The model under review builds one solid part; all positions refer to its coordinate system, in mm. Face numbers are marked on the shaded views. A direction names the side the tool comes from. Round coordinates to 2 decimals unless told otherwise and drop trailing zeros. Order: outer loops, then holes, each group sorted by start corner. A loop starts at its lowest first (then second) coordinate and runs counter-clockwise, first axis right, second up.
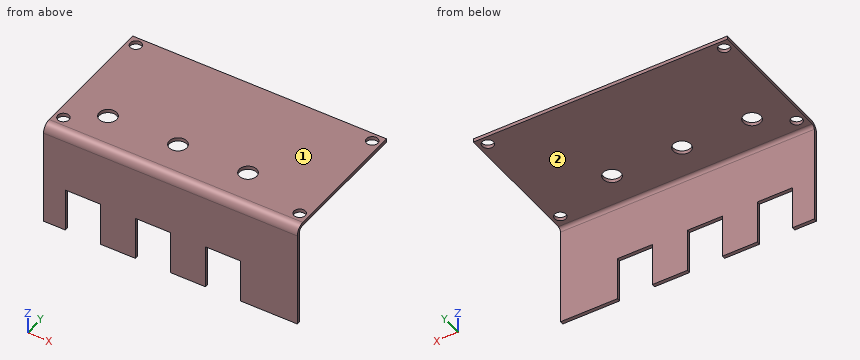
```python
from build123d import *

# Parameters (mm, degrees)
F1_DEPTH = 72.5
F2_W     = 20
F2_H     = 25
F3_DEPTH = 25
F4_R     = 5
F5_DEPTH = 25
F6_R     = 3.25
F7_DEPTH = 25


with BuildPart() as f1:
    # F0 (on Right) → F1 (new body, symmetric)
    with BuildSketch(Plane.YZ):
        with BuildLine():
            Line((34.471770674, 53.4658672512), (34.471770674, 55.4658672512))
            Line((34.471770674, 55.4658672512), (-40.528229326, 55.4658672512))
            ThreePointArc((-40.528229326, 55.4658672512), (-44.0637632319, 54.0014011571), (-45.528229326, 50.4658672512))
            Line((-45.528229326, 50.4658672512), (-45.528229326, -4.5341327488))
            Line((-45.528229326, -4.5341327488), (-43.528229326, -4.5341327488))
            Line((-43.528229326, -4.5341327488), (-43.528229326, 51.4658672512))
            ThreePointArc((-43.528229326, 51.4658672512), (-42.9424428884, 52.8800808135), (-41.528229326, 53.4658672512))
            Line((-41.528229326, 53.4658672512), (34.471770674, 53.4658672512))
        make_face()
    extrude(amount=F1_DEPTH, both=True)

    # F2 (on face) → F3 (cut)
    with BuildSketch(Plane.XZ.offset(45.528229326)):
        with Locations((-50, 7.9658672512)):
            Rectangle(F2_W, F2_H)
        with Locations((-10, 7.9658672512)):
            Rectangle(F2_W, F2_H)
        with Locations((30, 7.9658672512)):
            Rectangle(F2_W, F2_H)
    extrude(amount=-F3_DEPTH, mode=Mode.SUBTRACT)

    # F4 (on face) → F5 (cut)
    with BuildSketch(Plane.XY.offset(55.4658672512)):
        with Locations((-50, -23.028229326)):
            Circle(F4_R)
        with Locations((-10, -23.028229326)):
            Circle(F4_R)
        with Locations((30, -23.028229326)):
            Circle(F4_R)
    extrude(amount=-F5_DEPTH, mode=Mode.SUBTRACT)

    # F6 (on face) → F7 (cut)
    with BuildSketch(Plane.XY.offset(55.4658672512)):
        with Locations((-67.5, -35.528229326)):
            Circle(F6_R)
        with Locations((-67.5, 29.471770674)):
            Circle(F6_R)
        with Locations((67.5, 29.471770674)):
            Circle(F6_R)
        with Locations((67.5, -35.528229326)):
            Circle(F6_R)
    extrude(amount=-F7_DEPTH, mode=Mode.SUBTRACT)


solid = f1.part
```
(1) Consider section C-C (x = 67.5). Write out the cut boundary in (y, z).
Data:
outline: (-45.53, -4.53) - (-43.53, -4.53) - (-43.53, 51.47) arc R2 cw to (-41.53, 53.47) - (-38.78, 53.47) - (-38.78, 55.47) - (-40.53, 55.47) arc R5 ccw to (-45.53, 50.47) - close; (-32.28, 53.47) - (26.22, 53.47) - (26.22, 55.47) - (-32.28, 55.47) - close; (32.72, 53.47) - (34.47, 53.47) - (34.47, 55.47) - (32.72, 55.47) - close
(2) Consider section D-D (x = -26.5). Write out the cut boundary in (y, z).
Data:
outline: (-45.53, -4.53) - (-43.53, -4.53) - (-43.53, 51.47) arc R2 cw to (-41.53, 53.47) - (34.47, 53.47) - (34.47, 55.47) - (-40.53, 55.47) arc R5 ccw to (-45.53, 50.47) - close
(3) Insertion check: pin 1 (0.6 mm diameter, centred on x = -9, y = -44, fed in from -Z); pin 2 (4 mm diameter, centred on x = 67.5, y = -35.53, fed in from +Z); pin 3 (8 mm diameter, centred on x = -25.5, z = 4, fed in from +Y); pin 4 (10.5 mm diameter, centred on x = -67.5, y = 29.47, fed in from +Z). Each pin has a flat end and moves straight along its axis. Give the tip position at first contact, or say it passes through.
Data:
pin 1: stops at z = 20.47
pin 2: passes through
pin 3: stops at y = -43.53
pin 4: stops at z = 55.47
(4) Consider section A-A (x = 30). Write out the cut boundary in (y, z), and give its area (3 significant figures).
Data:
outline: (-45.53, 20.47) - (-43.53, 20.47) - (-43.53, 51.47) arc R2 cw to (-41.53, 53.47) - (-28.03, 53.47) - (-28.03, 55.47) - (-40.53, 55.47) arc R5 ccw to (-45.53, 50.47) - close; (-18.03, 53.47) - (34.47, 53.47) - (34.47, 55.47) - (-18.03, 55.47) - close
area: 201 mm2
(5) For the marked faces 1 and 2, list the 3-axis set-ups (+Z, -Z, +X, -X, +Y, -Y) from which the entire face can be reached by the end or side of a thin tool; tool diameter is ignored.
Data:
face 1: +Z, +X, -X, +Y, -Y
face 2: -Z, +X, -X, +Y
(6) To check wall thickness, follow probe 1 along Y at (x, z) = (-50, 54.45); probe 2 along Y at (x, z) = (-67.5, 54.15); probe 3 along Z at (x, y) = (28, -17). State the ranges of each line that lie inside material, in increasing order.
Data:
probe 1: y = -43.55 to -28.03, -18.03 to 34.47
probe 2: y = -43.91 to -38.78, -32.28 to 26.22, 32.72 to 34.47
probe 3: z = 53.47 to 55.47
(7) Consider section B-B (z = 9). Write out the cut boundary in (x, y).
Data:
outline: (-72.5, -45.53) - (-60, -45.53) - (-60, -43.53) - (-72.5, -43.53) - close; (-40, -45.53) - (-20, -45.53) - (-20, -43.53) - (-40, -43.53) - close; (0, -45.53) - (20, -45.53) - (20, -43.53) - (0, -43.53) - close; (40, -45.53) - (72.5, -45.53) - (72.5, -43.53) - (40, -43.53) - close
